from build123d import *

# Parameters (mm, degrees)
SKETCH2_W           = 30
SKETCH2_H           = 30
BOSS_EXTRUDE1_DEPTH = 100
CUT_EXTRUDE1_START  = -30
CUT_EXTRUDE1_DEPTH  = 30
CUT_EXTRUDE2_DEPTH  = 69
CUT_EXTRUDE3_DEPTH  = 72.7


# Read off the part's stored shape, not the designer's step: Cut-Extrude1
with BuildPart() as part:
    # Sketch2 → Boss-Extrude1 (new body)
    with BuildSketch(Plane.XY):
        with Locations((-15, 15)):
            Rectangle(SKETCH2_W, SKETCH2_H)
    extrude(amount=BOSS_EXTRUDE1_DEPTH)

    # Cut-Extrude1 outline → Cut-Extrude1 (cut)
    with BuildSketch(Plane.XZ.offset(CUT_EXTRUDE1_START)):
        with BuildLine():
            ThreePointArc((-30, 69.824648593), (-16.445900415, 82.511221459), (0, 91.124879576))
            Line((0, 91.124879576), (0, 100))
            Line((0, 100), (-30, 100))
            Line((-30, 100), (-30, 69.824648593))
        make_face()
    extrude(amount=CUT_EXTRUDE1_DEPTH, mode=Mode.SUBTRACT)

    # Sketch4 → Cut-Extrude2 (cut)
    with BuildSketch(Plane(origin=(0, 0, 0), x_dir=(-1, 0, 0), z_dir=(0, 0, -1))):
        with BuildLine():
            Line((3, 15), (0, 15))
            Line((0, 15), (0, 30))
            Line((0, 30), (30, 30))
            Line((30, 30), (30, 15))
            Line((30, 15), (27, 15))
            ThreePointArc((27, 15), (15, 3), (3, 15))
        make_face()
    extrude(amount=-CUT_EXTRUDE2_DEPTH, mode=Mode.SUBTRACT)

    # Sketch5 → Cut-Extrude3 (cut)
    with BuildSketch(Plane(origin=(0, 0, 0), x_dir=(-1, 0, 0), z_dir=(0, 0, -1))):
        Polygon((0, 0), (0, 10), (10, 0), align=None)
    extrude(amount=-CUT_EXTRUDE3_DEPTH, mode=Mode.SUBTRACT)


solid = part.part
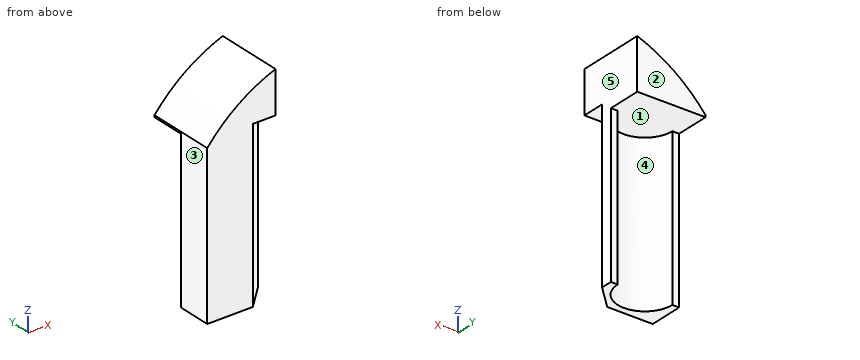
Work out the finished part from the listing and answer in its coordinate system (mm). Face numbers are marked on the shaded views. A direction names the side the tool comes from. Coordinates: 2 decimals unless noted, no trailing zeros. Loops run counter-clockwise (first coordinate to the right, second up) from the corner with the lowest first, then second, coordinate; pieces in that order, holes last. Notation, with made-up numbers: (43.25, 40) -> (94.25, 40) arc R27 cw to (94.25, 76) -> close; hole circle Ø6 at (32, 59). An arc over 180 degrees is marked (long way). Answer as CSV lines item,"result".
1) For a pull along X with two mould halves and no side action, classify the marked faces 1, 2 and 3 as released by +X, released by -X, zero draft, split by the parting line, or undercut.
A:
face 1,"undercut"
face 2,"zero draft"
face 3,"released by -X"
2) The part is cut by section A-A (z = 18.5). Give the vertices of the cut face in (x, y).
A:
outline,"(-30, 0) -> (-10, 0) -> (0, 10) -> (0, 15) -> (-3, 15) arc R12 cw to (-27, 15) -> (-30, 15) -> close"
3) Flat-ended cylindrical pins translate along their axes: pin 1 (8 mm diameter, centred on x = -15, y = 12.5, fed in from +Z); pin 2 (12 mm diameter, centred on x = -17.5, z = 20.5, fed in from +Y); pin 3 (2.5 mm diameter, centred on x = -1, z = 35.5, fed in from +Y). Find the tip coordinate at first contact, or state that the pin passes through.
A:
pin 1,"stops at z = 86.01"
pin 2,"stops at y = 6.53"
pin 3,"stops at y = 15"
4) The part is cut by section C-C (y = 8). Give the vertices of the cut face in (x, z).
A:
outline,"(-30, 0) -> (-24.75, 0) -> (-24.75, 69) -> (-5.25, 69) -> (-5.25, 0) -> (-2, 0) -> (-2, 72.7) -> (0, 72.7) -> (0, 91.12) arc R69 ccw to (-30, 69.82) -> close"
5) Straight lines are drawn through the part: probe 1 along Y at (x, z) = (-15.5, 33); probe 2 along X at (y, z) = (10, 41.5); probe 3 along X at (y, z) = (7.5, 24.5). For each, find the intervals that lie inside material, in ascending order.
A:
probe 1,"y = 0 to 3.01"
probe 2,"x = -30 to -25.91, -4.09 to 0"
probe 3,"x = -30 to -24.37, -5.63 to -2.5"
6) The part is cut by section D-D (x = -4.5). Give the vertices of the cut face in (y, z).
A:
outline,"(0, 72.7) -> (5.5, 72.7) -> (5.5, 0) -> (9.19, 0) -> (9.19, 69) -> (30, 69) -> (30, 89.31) -> (0, 89.31) -> close"
7) For the marked faces 4 and 5, determine the directions among +Z, -Z, +X, -X, +Y, -Y from which every point of the face is accessible in a straight line to the end or side of a thin tool.
A:
face 4,"-Z, +Y"
face 5,"+Z, -Z, +X, +Y, -Y"
8) The part is cut by section B-B (x = -15). Give the vertices of the cut face in (y, z), and give its area (3 significant figures).
A:
outline,"(0, 0) -> (3, 0) -> (3, 69) -> (30, 69) -> (30, 83.51) -> (0, 83.51) -> close"
area,"642 mm²"
